CAD build for the part. Positions are in the model's coordinates, mm. Round coordinates to 2 decimals unless told otherwise and drop trailing zeros. Write each loop counter-clockwise with the first axis right and the second up, starting at its lowest first coordinate (ties: lowest second). Pieces come first, ordered by that corner, then holes. Notation, with made-up numbers: (33.5, 4.5) - (82.5, 4.5) arc R15 ccw to (82.5, 18.5) - close; hole circle Ø3 at (52.5, 29.25). An arc over 180 degrees is marked (long way). Answer in a Markdown table with one row per item.
```python
from build123d import *

# Parameters (mm, degrees)
EXTRUDE_1_DEPTH   = 2
HOLE_WIZARD_M81_D = 9
CHAMFER_1_SIZE    = 2


with BuildPart() as part:
    # Эскиз1 → Бобышка-Вытянуть1 (new body)
    with BuildSketch(Plane(origin=(0, 0, 0), x_dir=(1, 0, 0), z_dir=(0, 0, -1))):
        Polygon((0, 0), (0, 120), (80, 120), (80, 80), (40, 80), (40, 0), align=None)
    extrude(amount=EXTRUDE_1_DEPTH)

    # Отверстие с зазором M81 (through all)
    with Locations(Plane(origin=(0, 0, -2), x_dir=(1, 0, 0), z_dir=(0, 0, -1))):
        with Locations((60, 100), (20, 100), (20, 60), (20, 20)):
            Hole(HOLE_WIZARD_M81_D / 2)

    # Фаска1
    chamfer_1_edges = [part.edges().sort_by_distance(p)[0] for p in [
        (0, 0, -1),
        (0, -120, -1),
        (80, -120, -1),
        (80, -80, -1),
        (40, 0, -1),
    ]]
    chamfer(chamfer_1_edges, length=CHAMFER_1_SIZE)


solid = part.part
```
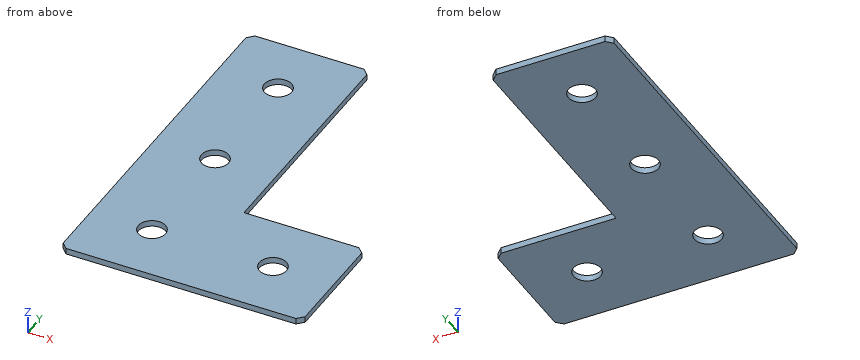
Q1. Drill centre lines: line 1 (Y direction, x = 20, z = -0.9); line 2 (X direction, y = -100, z = -0.95); line 3 (Y direction, x = 60, z = -0.65). Where is each one in solid material? Low to high.
Computed:
| item | result |
|---|---|
| line 1 | y = -120 to -104.5, -95.5 to -64.5, -55.5 to -24.5, -15.5 to 0 |
| line 2 | x = 0 to 15.5, 24.5 to 55.5, 64.5 to 80 |
| line 3 | y = -120 to -104.5, -95.5 to -80 |
Q2. Flat gauge pins, fed straight in: pin 1 (0.6 mm diameter, centred on y = -50, z = -0.5, fed in from +X); pin 2 (5.5 mm diameter, centred on x = 20, y = -20, fed in from -Z). Where does each tip first touch, or does it go through?
Computed:
| item | result |
|---|---|
| pin 1 | stops at x = 40 |
| pin 2 | passes through |
Q3. Saw through at B-B on y = -20. List the corners of the cut face in (x, z), then the cut area to 3 significant figures.
Computed:
| item | result |
|---|---|
| outline | (0, -2) - (15.5, -2) - (15.5, 0) - (0, 0) - close; (24.5, -2) - (40, -2) - (40, 0) - (24.5, 0) - close |
| area | 62.0 mm2 |
Q4. Saw through at C-C on x = 20. List the corners of the cut face in (y, z).
Computed:
| item | result |
|---|---|
| outline | (-120, -2) - (-104.5, -2) - (-104.5, 0) - (-120, 0) - close; (-95.5, -2) - (-64.5, -2) - (-64.5, 0) - (-95.5, 0) - close; (-55.5, -2) - (-24.5, -2) - (-24.5, 0) - (-55.5, 0) - close; (-15.5, -2) - (0, -2) - (0, 0) - (-15.5, 0) - close |
Q5. Saw through at D-D on y = -100. List the corners of the cut face in (x, z), then the cut area to 3 significant figures.
Computed:
| item | result |
|---|---|
| outline | (0, -2) - (15.5, -2) - (15.5, 0) - (0, 0) - close; (24.5, -2) - (55.5, -2) - (55.5, 0) - (24.5, 0) - close; (64.5, -2) - (80, -2) - (80, 0) - (64.5, 0) - close |
| area | 124 mm2 |
Q6. Saw through at A-A on x = 60. List the corners of the cut face in (y, z).
Computed:
| item | result |
|---|---|
| outline | (-120, -2) - (-104.5, -2) - (-104.5, 0) - (-120, 0) - close; (-95.5, -2) - (-80, -2) - (-80, 0) - (-95.5, 0) - close |
